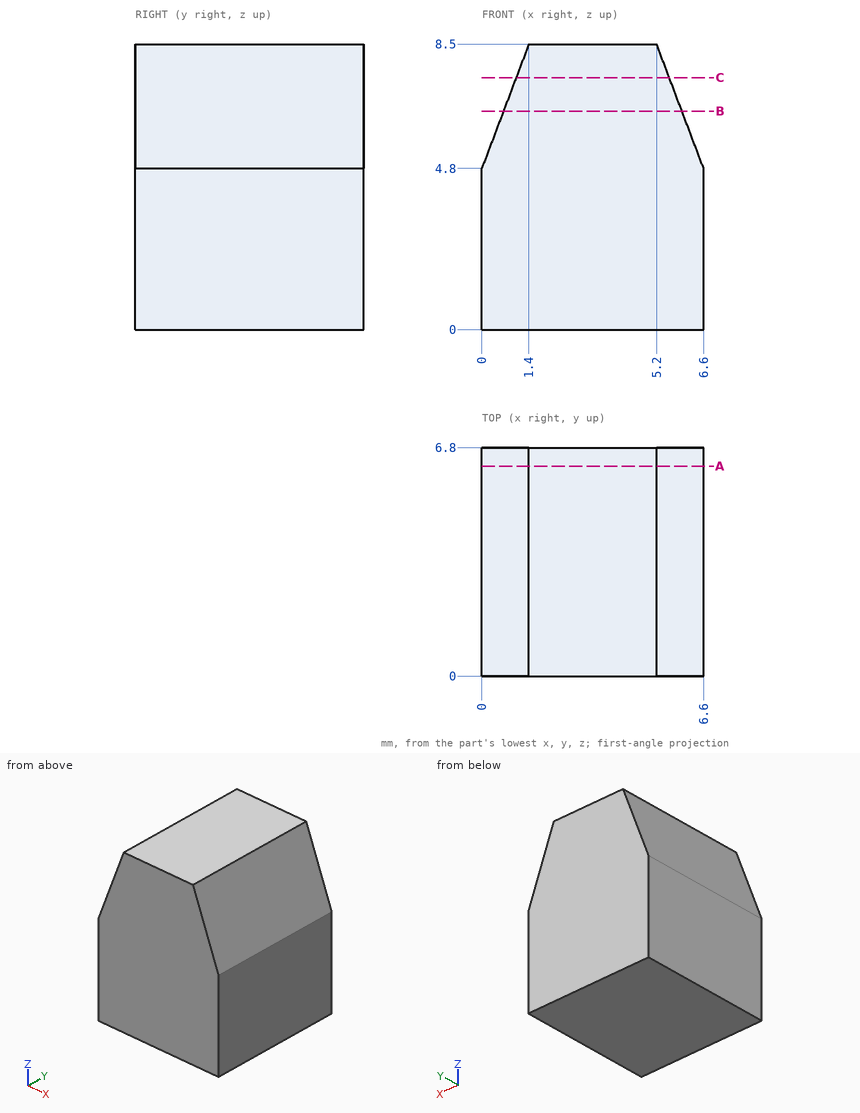
Study the drawing (mm; zero at the part's minimum x, y, z) and answer. Coordinates: 2 decimals unless noted, no trailing zeros. Loops run counter-clockwise (first coordinate to the right, second up) from the corner with the lowest first, then second, coordinate; pieces in that order, holes last. Notation, with made-up numbers: M 57,-38.75 L 108,-38.75 A23 ccw 108,-7.75 Z; hole C -31,-33.5 d2. An arc over 180 degrees is marked long. Answer as a JSON object with one key per item and string values. Group by question number.
Item 1: Section B-B (z = 6.5) is taken. Write down the section's boundary in (x, y).
Item 2: Section A-A (y = 6.25) is taken. Write down the section's boundary in (x, z), and give its area (3 significant figures).
Item 3: Section C-C (z = 7.5) is taken. Write down the section's boundary in (x, y).
Item 4: Consider L1, parallel to X at y = 6, z = 5; L2, parallel to X at y = 4.5, z = 6.25. Determine where each line is inside the solid, lowest interval first.
Solved:
{
 "1": {"outline": "M 0.64,0 L 5.96,0 L 5.96,6.8 L 0.64,6.8 Z"},
 "2": {"outline": "M 0,0 L 6.6,0 L 6.6,4.8 L 5.2,8.5 L 1.4,8.5 L 0,4.8 Z", "area": "50.9 mm2"},
 "3": {"outline": "M 1.02,0 L 5.58,0 L 5.58,6.8 L 1.02,6.8 Z"},
 "4": {"L1": "x = 0.08 to 6.52", "L2": "x = 0.55 to 6.05"}
}
